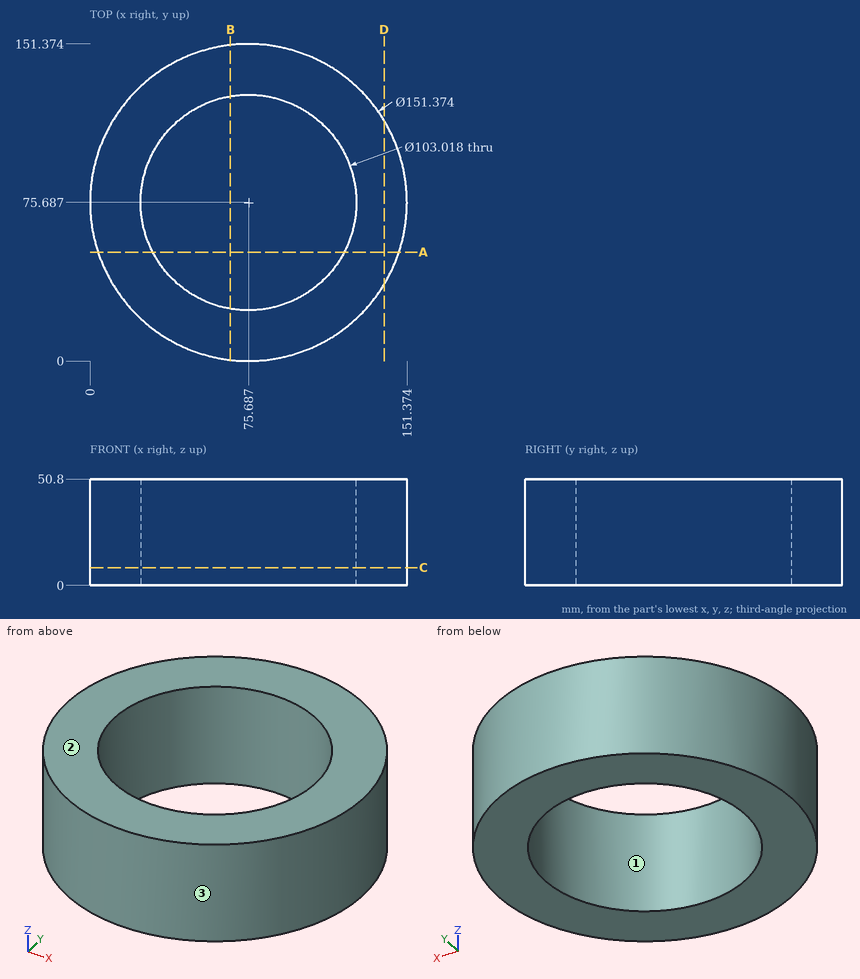
Verification items for this drawing (mm, ordinates from the low corner). Coordinates: 2 decimals unless noted, no trailing zeros. Order: outer loops, then holes, each group sorted by start corner. A loop starts at its lowest first (then second) coordinate and runs counter-clockwise, first axis right, second up. Notation, with made-up numbers: (13, 21) -> (29, 21) arc R25 ccw to (29, 44) -> close; hole circle Ø8 at (-38.75, 39.25). An arc over 180 degrees is marked (long way). Answer as CSV lines item,"result". Start each with the question number.
1) Cross-section at A-A, the plane y = 52. Record the boundary of the cut face in (x, z), then the cut area to 3 significant figures.
2) Release check for a two-part mould opening along X. For the marked faces 1, 2 and 3 record: released by +X, released by -X, zero draft, split by the parting line, or undercut.
3) Gauge pin test, flat ends, axial feed: pin 1 Ø2 at (y, z) = (23.5, 7.5) entering from +X; pin 2 Ø1.5 at (y, z) = (32, 24.5) entering from -X; pin 3 Ø3 at (y, z) = (117.5, 23) entering from +X. Record the tip position at first contact, or that the pin passes through.
4) Cross-section at D-D, the plane x = 140.5. Record the boundary of the cut face in (y, z).
5) Cross-section at B-B, the plane x = 67. Record the boundary of the cut face in (y, z), then the cut area to 3 significant figures.
6) Cross-section at C-C, the plane z = 8.5. Record the boundary of the cut face in (x, y), then the cut area to 3 significant figures.
7) Material ranges on L1, parallel to X at y = 36.5, z = 25 (1 decimal); L2, parallel to X at y = 112.5, z = 12 (1 decimal); L3, parallel to Y at x = 59.5, z = 21.5, recorded low to high. Write a range as [from, to].
Conclusion:
1,outline,"(3.8, 0) -> (29.95, 0) -> (29.95, 50.8) -> (3.8, 50.8) -> close; (121.43, 0) -> (147.57, 0) -> (147.57, 50.8) -> (121.43, 50.8) -> close"
1,area,"2,660 mm²"
2,face 1,"undercut"
2,face 2,"zero draft"
2,face 3,"split by the parting line"
3,pin 1,"stops at x = 131.44"
3,pin 2,"stops at x = 13.36"
3,pin 3,"stops at x = 139.74"
4,outline,"(36.6, 0) -> (114.77, 0) -> (114.77, 50.8) -> (36.6, 50.8) -> close"
5,outline,"(0.5, 0) -> (24.92, 0) -> (24.92, 50.8) -> (0.5, 50.8) -> close; (126.46, 0) -> (150.87, 0) -> (150.87, 50.8) -> (126.46, 50.8) -> close"
5,area,"2,480 mm²"
6,outline,"circle Ø151.37 at (75.69, 75.69); hole circle Ø103.02 at (75.69, 75.69)"
6,area,"9,660 mm²"
7,L1,"x = [10.9, 42.3], [109.1, 140.4]"
7,L2,"x = [9.6, 39.7], [111.7, 141.8]"
7,L3,"y = [1.75, 26.79], [124.59, 149.62]"
